Read the model definition and answer for the solid it produces. Units are mm, in the model's axes. A direction names the side the tool comes from. Coordinates: 2 decimals unless noted, no trailing zeros. Order: outer loops, then holes, each group sorted by start corner. A loop starts at its lowest first (then second) coordinate and runs counter-clockwise, first axis right, second up. Notation, with made-up numbers: (-21.75, 54) -> (1.25, 54) arc R12 cw to (1.25, 62) -> close; hole circle Ø3 at (69.5, 24). An arc over 180 degrees is marked (long way). Answer as a JSON object with one key per item and string values. Group by question number.
1) A tool of negligible diameter and unlimited length cuts with its end or side. For faces 4 (the flat face through (0, -45, 1)), 5 (the flat face through (7, -22, 25)), 6 (the flat face through (0, -41.5, 8)), 7 (the flat face through (0, -1.5, 8)), 8 (the cylindrical face through (-4.3, -21.92, 29.05)), from which of +Z, -Z, +X, -X, +Y, -Y can it reach the whole face along a straight path? Write none if from no direction.
2) Section B-B on y = -45.5 is taken. Determine the outline of the cut face in (x, z).
3) Section A-A on y = -24.2 is taken. Determine the outline of the cut face in (x, z).
4) Given pin 1 (6.5 mm diameter, centred on x = -5, y = -45.5, fed in from +Z); pin 2 (2.5 mm diameter, centred on x = -1.5, y = 0.5, fed in from -Z); pin 3 (0.6 mm diameter, centred on y = -20.5, z = 24, fed in from +X), each flat-ended and moving along its own axis, determine where each tip first touches the part or whether it passes through.
5) Consider L1, parallel to X at y = 2.5, z = 2.8; L2, parallel to X at y = -45, z = 2; L3, parallel to Z at x = 8.75, y = -10. Determine where each line is inside the solid, lowest interval first.
6) Determine the mould class of faces 1 (the flat face through (0, -1.5, -13)), 2 (the cylindrical face through (4.9, -21.92, 29.05)), 3 (the cylindrical face through (-6.983, 2.24, 2.268)) for opening direction Y: released by +Y, released by -Y, zero draft, split by the parting line, or undercut.
7) Section C-C on x = 0 is taken. Determine the outline of the cut face in (y, z).
8) Section D-D on z = 22.5 is taken. Determine the outline of the cut face in (x, y), and give its area (3 significant figures).
from build123d import *

# Parameters (mm, degrees)
CYLINDER001_R             = 2
CYLINDER001_DEPTH         = 10
CYLINDER_R                = 2
CYLINDER_DEPTH            = 10
BOX001_W                  = 7.6
BOX001_H                  = 20
BOX001_DEPTH              = 2.5
BOX_W                     = 40
BOX_H                     = 20
BOX_DEPTH                 = 39
BOX002_W                  = 14
BOX002_H                  = 16
BOX002_DEPTH              = 2
CYLINDER002_R             = 9
CYLINDER002_DEPTH         = 13
CYLINDER004_R             = 2.3
CYLINDER004_DEPTH         = 7
CYLINDER003_R             = 2.3
CYLINDER003_DEPTH         = 7
FUSION009_PLACEMENT_ANGLE = 90
BODY_ROLL_ANGLE           = 180
BODY_PLACEMENT_ANGLE      = -90


with BuildPart() as cylinder001:
    # Cylinder001 → Cylinder001 (new body)
    with BuildSketch(Plane(origin=(44, 15, 5), x_dir=(1, 0, 0), z_dir=(0, 0, 1))):
        Circle(CYLINDER001_R)
    extrude(amount=CYLINDER001_DEPTH)


with BuildPart() as fusion:
    # Cylinder → Cylinder (new body)
    with BuildSketch(Plane(origin=(44, 5, 5), x_dir=(1, 0, 0), z_dir=(0, 0, 1))):
        Circle(CYLINDER_R)
    extrude(amount=CYLINDER_DEPTH)

    # Fusion: union Cylinder001
    add(cylinder001.part)


with BuildPart() as cut:
    # Box001 → Box001 (new body)
    with BuildSketch(Plane(origin=(40, 0, 9), x_dir=(1, 0, 0), z_dir=(0, 0, 1))):
        with Locations((3.8, 10)):
            Rectangle(BOX001_W, BOX001_H)
    extrude(amount=BOX001_DEPTH)

    # Cut: cut Fusion
    add(fusion.part, mode=Mode.SUBTRACT)


with BuildPart() as cut_1:
    # Cut placement: moved
    add(cut.part.moved(Location((-10, -10, 0))))


with BuildPart() as part_mirroring:
    # Part__Mirroring: instance of Cut
    add(cut_1.part.mirror(Plane(origin=(0, 0, 0), x_dir=(0, -1, 0), z_dir=(1, 0, 0))))


with BuildPart() as part_mirroring_1:
    # Part__Mirroring placement: moved
    add(part_mirroring.part.moved(Location((20, 0, 0))))


with BuildPart() as fusion010:
    # Box → Box (new body)
    with BuildSketch(Plane(origin=(-10, -10, 0), x_dir=(1, 0, 0), z_dir=(0, 0, 1))):
        with Locations((20, 10)):
            Rectangle(BOX_W, BOX_H)
    extrude(amount=BOX_DEPTH)

    # Fusion010: union Part__Mirroring, Cut
    add(part_mirroring_1.part)
    add(cut_1.part)


with BuildPart() as cube002:
    # Box002 → Box002 (new body)
    with BuildSketch(Plane(origin=(-7, -15, 0), x_dir=(1, 0, 0), z_dir=(0, 0, 1))):
        with Locations((7, 8)):
            Rectangle(BOX002_W, BOX002_H)
    extrude(amount=BOX002_DEPTH)


with BuildPart() as shaft:
    # Cylinder002 → Cylinder002 (new body)
    with BuildSketch(Plane.XY):
        Circle(CYLINDER002_R)
    extrude(amount=CYLINDER002_DEPTH)


with BuildPart() as cylinder004:
    # Cylinder004 → Cylinder004 (new body)
    with BuildSketch(Plane(origin=(4.6, -12.7, -7), x_dir=(1, 0, 0), z_dir=(0, 0, 1))):
        Circle(CYLINDER004_R)
    extrude(amount=CYLINDER004_DEPTH)


with BuildPart() as servo:
    # Cylinder003 → Cylinder003 (new body)
    with BuildSketch(Plane(origin=(-4.6, -12.7, -7), x_dir=(1, 0, 0), z_dir=(0, 0, 1))):
        Circle(CYLINDER003_R)
    extrude(amount=CYLINDER003_DEPTH)

    # Fusion009: union Cube002, shaft, Cylinder004
    add(cube002.part)
    add(shaft.part)
    add(cylinder004.part)


with BuildPart() as servo_1:
    # Fusion009 placement: moved
    add(servo.part.moved(Location((0, 0, -13))).rotate(Axis((0, 0, -13), (0, 0, 1)), FUSION009_PLACEMENT_ANGLE))

    # Fusion011: union Fusion010
    add(fusion010.part)


with BuildPart() as servo_2:
    # Fusion011 placement: moved
    add(servo_1.part.moved(Location((10, 10, 0))))


with BuildPart() as servo_3:
    # Body roll: moved
    add(servo_2.part.rotate(Axis((0, 0, 0), (1, 0, 0)), BODY_ROLL_ANGLE))


with BuildPart() as servo_4:
    # Body placement: moved
    add(servo_3.part.moved(Location((10, -1.5, 12.5))).rotate(Axis((10, -1.5, 12.5), (0, 0, 1)), BODY_PLACEMENT_ANGLE))


solid = servo_4.part
Worked answers:
{
 "1": {"face 4": "-Z, +X, -X, -Y", "face 5": "+Z, +X, -Y", "face 6": "+Z, +X, -X, -Y", "face 7": "+Z, +X, -X, +Y", "face 8": "+Z"},
 "2": {"outline": "(-10, 1) -> (-7, 1) -> (-7, 3.5) -> (-10, 3.5) -> close; (-3, 1) -> (3, 1) -> (3, 3.5) -> (-3, 3.5) -> close; (7, 1) -> (10, 1) -> (10, 3.5) -> (7, 3.5) -> close"},
 "3": {"outline": "(-10, -26.5) -> (10, -26.5) -> (10, 12.5) -> (-10, 12.5) -> close; (-7, 23.5) -> (7, 23.5) -> (7, 25.5) -> (6.9, 25.5) -> (6.9, 32.5) -> (2.3, 32.5) -> (2.3, 25.5) -> (-2.3, 25.5) -> (-2.3, 32.5) -> (-6.9, 32.5) -> (-6.9, 25.5) -> (-7, 25.5) -> close"},
 "4": {"pin 1": "stops at z = 3.5", "pin 2": "stops at z = 1", "pin 3": "stops at x = 7"},
 "5": {"L1": "x = -10 to -7, -3 to 3, 7 to 10", "L2": "x = -10 to -6.94, -3.06 to 3.06, 6.94 to 10", "L3": "z = -26.5 to 25.5"},
 "6": {"face 1": "released by +Y", "face 2": "split by the parting line", "face 3": "undercut"},
 "7": {"outline": "(-49.1, 1) -> (-41.5, 1) -> (-41.5, -26.5) -> (-1.5, -26.5) -> (-1.5, 1) -> (6.1, 1) -> (6.1, 3.5) -> (-1.5, 3.5) -> (-1.5, 12.5) -> (-2.5, 12.5) -> (-2.5, 25.5) -> (-26.5, 25.5) -> (-26.5, 23.5) -> (-20.5, 23.5) -> (-20.5, 12.5) -> (-41.5, 12.5) -> (-41.5, 3.5) -> (-49.1, 3.5) -> close"},
 "8": {"outline": "circle Ø18 at (0, -11.5)", "area": "254 mm²"}
}
